Could you check a few things on this model? Use its own coordinates, in mm. Face numbers are marked on the shaded views. A direction names the side the tool comes from. Give positions to 0.01 mm unless a question says otherwise; leave off trailing zeros. Loops run counter-clockwise (first coordinate to the right, second up) from the corner with the lowest first, then second, coordinate; pieces in that order, holes last. Notation, with made-up numbers: (55, -19.75) - (111, -19.75) arc R22 ccw to (111, 9.25) - close; hole circle Ø5 at (-14.75, 76.5). An arc over 180 degrees is marked (long way). One line per item, written item: value. Start each with the question number.
Q1. If we mould it in two halves opening along X, with no side actions, what happens to the marked faces 1, 2, 3 and 4? For each: released by +X, released by -X, zero draft, split by the parting line, or undercut.
Q2. If I drill on line 1 (X direction, y = 2, z = -4); line 2 (Y direction, x = -0.25, z = 2.5), over which ranges is the centre line in solid material (lowest first)? Write a range as from..to.
Q3. I'm going to push a flat-ended pin straight in: P1, Ø3, axis at x = 3.5, z = 1, coming from the -Y side. Where does the tip first touch, or does it pass through?
Q4. For the marked faces 5 and 6, which set-ups out of +Z, -Z, +X, -X, +Y, -Y let a thin tool reach every point of the face, with its end or its side?
Q5. I want a section at C-C (x = 8). Please give me the cut outline in (y, z).
Q6. I want a section at A-A (y = 2). Please give me the cut outline in (x, z).
Q7. I want a section at B-B (z = -4.5). Please give me the cut outline in (x, y), then the cut area to 3 significant figures.
```python
from build123d import *

# Parameters (mm, degrees)
SKETCH1_W           = 21
SKETCH1_H           = 10
BOSS_EXTRUDE1_DEPTH = 7
SKETCH2_W           = 17
SKETCH2_H           = 5
CUT_EXTRUDE1_DEPTH  = 10


with BuildPart() as part:
    # Sketch1 → Boss-Extrude1 (new body)
    with BuildSketch(Plane(origin=(0, 0, 0), x_dir=(1, 0, 0), z_dir=(0, 1, 0))):
        with Locations((2.759910232, 1.119822485)):
            Rectangle(SKETCH1_W, SKETCH1_H)
    extrude(amount=BOSS_EXTRUDE1_DEPTH)

    # Sketch2 → Cut-Extrude1 (cut)
    with BuildSketch(Plane.XY.offset(3.880177515)):
        with Locations((2.759910232, 2.5)):
            Rectangle(SKETCH2_W, SKETCH2_H)
    extrude(amount=-CUT_EXTRUDE1_DEPTH, mode=Mode.SUBTRACT)


solid = part.part
```
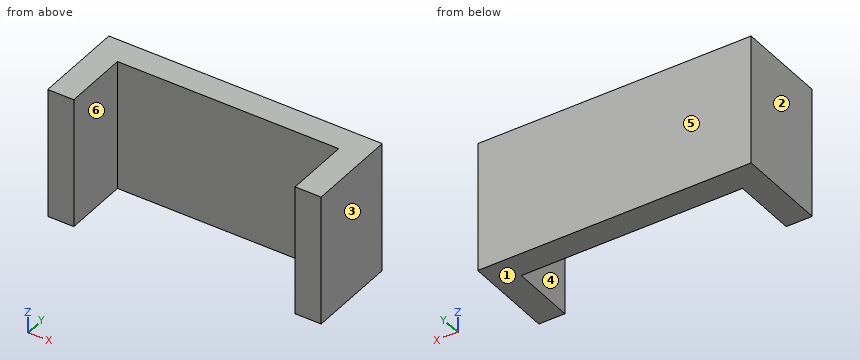
Worked answers:
1. face 1: zero draft
1. face 2: released by -X
1. face 3: released by +X
1. face 4: undercut
2. line 1: x = -7.74..-5.74, 11.26..13.26
2. line 2: y = 5..7
3. P1: stops at y = 5
4. face 5: +Z, -Z, +X, -X, +Y
4. face 6: +Z, -Z, -Y
5. outline: (5, -6.12) - (7, -6.12) - (7, 3.88) - (5, 3.88) - close
6. outline: (-7.74, -6.12) - (-5.74, -6.12) - (-5.74, 3.88) - (-7.74, 3.88) - close; (11.26, -6.12) - (13.26, -6.12) - (13.26, 3.88) - (11.26, 3.88) - close
7. outline: (-7.74, 0) - (-5.74, 0) - (-5.74, 5) - (11.26, 5) - (11.26, 0) - (13.26, 0) - (13.26, 7) - (-7.74, 7) - close
7. area: 62.0 mm²
